```python
from build123d import *

# Parameters (mm, degrees)
SKETCH1_R               = 3
BOSS_EXTRUDE1_DEPTH     = 14.5
BOSS_EXTRUDE2_DEPTH     = 2
CUT_EXTRUDE1_DEPTH      = 16.981969007
CUT_EXTRUDE1_DEPTH_BACK = 16.981969007


with BuildPart() as part:
    # Sketch1 → Boss-Extrude1 (new body)
    with BuildSketch(Plane(origin=(0, 0, 0), x_dir=(1, 0, 0), z_dir=(0, 1, 0))):
        with Locations(Location((0, 0, 0), (0, 0, 90))):
            Circle(SKETCH1_R)
    extrude(amount=BOSS_EXTRUDE1_DEPTH)

    # Sketch3 → Boss-Extrude2 (add)
    with BuildSketch(Plane(origin=(0, 0, 0), x_dir=(-1, 0, 0), z_dir=(0, -1, 0))):
        Polygon((5.080682369, 0), (2.540341184, 4.4), (-2.540341184, 4.4), (-5.080682369, 0), (-2.540341184, -4.4), (2.540341184, -4.4), align=None)
    extrude(amount=-BOSS_EXTRUDE2_DEPTH)

    # Sketch4 → Cut-Extrude1 (cut, two sides: drawn at the far end of the back side and taken through both)
    with BuildSketch(Plane(origin=(0, 14.5, 0), x_dir=(1, 0, 0), z_dir=(0, 1, 0)).offset(-CUT_EXTRUDE1_DEPTH_BACK)):
        with BuildLine():
            Line((-1.6, 0), (-1.6, -4.4))
            Line((-1.6, -4.4), (1.6, -4.4))
            Line((1.6, -4.4), (1.6, 0))
            ThreePointArc((1.6, 0), (0, 1.6), (-1.6, 0))
        make_face()
    extrude(amount=CUT_EXTRUDE1_DEPTH + CUT_EXTRUDE1_DEPTH_BACK, mode=Mode.SUBTRACT)


solid = part.part
```
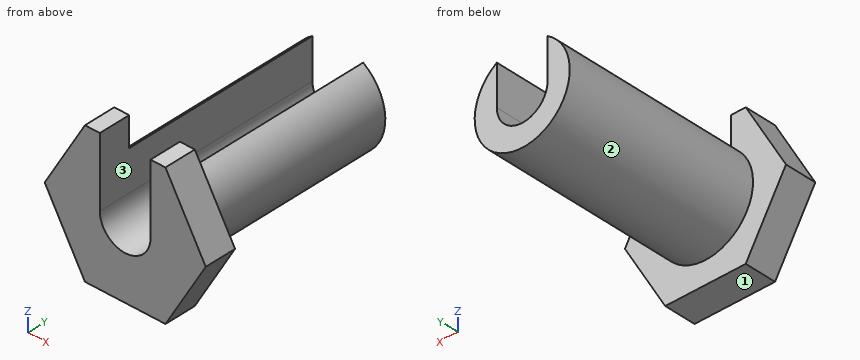
Geometry: final body of the model. Coordinates: model frame, mm. Face numbers are marked on the shaded views. A direction names the side the tool comes from. Coordinates: 2 decimals unless noted, no trailing zeros. Order: outer loops, then holes, each group sorted by start corner. A loop starts at its lowest first (then second) coordinate and runs counter-clockwise, first axis right, second up. Notation, with made-up numbers: (0, -36.5) -> (31, -36.5) arc R15 ccw to (31, -25.5) -> close; hole circle Ø6 at (-15.5, 79). An arc over 180 degrees is marked (long way). Answer in a Markdown table with one row per item.
Item 1: Section A-A on x = 0. Output: boundary loops of the cut face in (y, z), plus the area to 3 significant figures.
Return value:
| item | result |
|---|---|
| outline | (0, -4.4) -> (2, -4.4) -> (2, -3) -> (14.5, -3) -> (14.5, -1.6) -> (0, -1.6) -> close |
| area | 23.1 mm² |
Item 2: Section C-C on y = 1. Output: boundary loops of the cut face in (x, z).
Return value:
| item | result |
|---|---|
| outline | (-5.08, 0) -> (-2.54, -4.4) -> (2.54, -4.4) -> (5.08, 0) -> (2.54, 4.4) -> (1.6, 4.4) -> (1.6, 0) arc R1.6 cw to (-1.6, 0) -> (-1.6, 4.4) -> (-2.54, 4.4) -> close |
Item 3: Access query for the marked faces 1, 2 and 3. Directions: +Z, -Z, +X, -X, +Y, -Y. A direction counts if a zero-diameter tool reaches every point of the face in a straight line with its end or side. Return the directions, or none.
Return value:
| item | result |
|---|---|
| face 1 | -Z, +X, -X, +Y, -Y |
| face 2 | +Y |
| face 3 | +Z, +Y, -Y |
Item 4: Section B-B on z = 4. Output: boundary loops of the cut face in (x, y).
Return value:
| item | result |
|---|---|
| outline | (-2.77, 0) -> (-1.6, 0) -> (-1.6, 2) -> (-2.77, 2) -> close; (1.6, 0) -> (2.77, 0) -> (2.77, 2) -> (1.6, 2) -> close |
Item 5: Contact query for flat-ended pins moving along their axis: P1, Ø2, axis at x = 2.5, y = 6.5, coming from the -Z side; P2, Ø2, axis at y = 12.5, z = -2.5, coming from the -X side; P3, Ø2, axis at x = 2.5, y = 12, coming from the +Z side. Output: stop coordinate, or through.
Return value:
| item | result |
|---|---|
| P1 | stops at z = -2.6 |
| P2 | stops at x = -2.6 |
| P3 | stops at z = 2.54 |
Item 6: Ray query, L1, parallel to X at y = 12.5, z = 0; L2, parallel to X at y = 4.25, z = 2; L3, parallel to Y at x = 4.5, z = 0.5. Return the intervals inside material, ascending.
Return value:
| item | result |
|---|---|
| L1 | x = -3 to -1.6, 1.6 to 3 |
| L2 | x = -2.24 to -1.6, 1.6 to 2.24 |
| L3 | y = 0 to 2 |
Item 7: Section D-D on z = -2.5. Output: boundary loops of the cut face in (x, y).
Return value:
| item | result |
|---|---|
| outline | (-3.64, 0) -> (3.64, 0) -> (3.64, 2) -> (1.66, 2) -> (1.66, 14.5) -> (-1.66, 14.5) -> (-1.66, 2) -> (-3.64, 2) -> close |
